The model under review builds one solid part; all positions refer to its coordinate system, in mm. Face numbers are marked on the shaded views. A direction names the side the tool comes from. Coordinates: 2 decimals unless noted, no trailing zeros. Order: outer loops, then holes, each group sorted by start corner. A loop starts at its lowest first (then second) coordinate and runs counter-clockwise, first axis right, second up. Notation, with made-up numbers: M 81,29.5 L 94,29.5 A15 cw 94,56.5 Z; hole C 85,69.25 d9. An arc over 180 degrees is marked long. Answer as CSV lines item,"result". Start each with the question number.
Q1. Wall thickness on L1, parallel to X at y = 0.8, z = 5; L2, parallel to X at y = 24.5, z = 3.75; L3, parallel to X at y = 26.6, z = 0: over which ranges is each line inside the solid? List them lowest first. Write a range as [from, to].
Q2. Consider section D-D on z = 0. Write out the cut boundary in (x, y).
Q3. Consider section C-C on y = 23. Write out the cut boundary in (x, z), and give its area (3 significant figures).
Q4. Consider section B-B on x = -24.3. Write out the cut boundary in (y, z), and give its area (3 significant figures).
Q5. Consider section A-A on x = 9.3. Write out the cut boundary in (y, z), and give its area (3 significant figures).
Q6. The part is to be moulded in two halves that separate along X. For the marked faces 1, 2, 3 and 4, say which applies: +X half, -X half, draft (parallel to the pull), parting line (faces both ways), or undercut.
Q7. Machinability: for the marked faces 5 and 6, which of the approach directions +Z, -Z, +X, -X, +Y, -Y give a long, thin tool a straight path to every point of the face, cutting with its end or side? Answer none if there is none.
Q8. For P1, Ø1.8, axis at x = -24.3, z = 5, coming from the -Y side; P2, Ø1.8, axis at x = -24.5, y = 3.5, coming from the -Z side; P3, Ø6.5, axis at x = 23, y = 5.5, coming from the +Z side, all flat-tipped, find the tip position at first contact; note any pin that passes through.
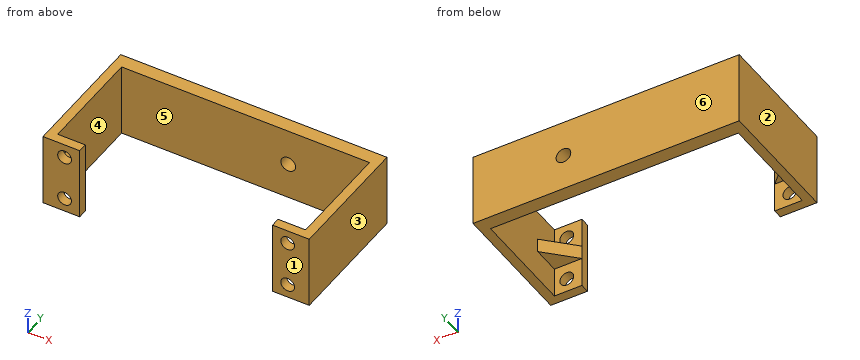
from build123d import *

# Parameters (mm, degrees)
RESSALTO_EXTRUS_O1_DEPTH = 8
ESBO_O2_R                = 1.5
CORTE_EXTRUS_O1_DEPTH    = 16
RESSALTO_EXTRUS_O3_DEPTH = 1.5
ESBO_O6_R                = 1.6
CORTE_EXTRUS_O2_DEPTH    = 3


with BuildPart() as part:
    # Esboço1 → Ressalto-extrusão1 (new, symmetric)
    with BuildSketch(Plane.XY):
        Polygon((-21, 0), (-29, 0), (-29, 28), (29, 28), (29, 0), (21, 0), (21, 2), (27, 2), (27, 25), (-27, 25), (-27, 2), (-21, 2), align=None)
    extrude(amount=RESSALTO_EXTRUS_O1_DEPTH, both=True)

    # Esboço2 → Corte-extrusão1 (cut)
    with BuildSketch(Plane.XZ):
        with Locations(Location((-24.3, -5, 0), (0, 0, 270))):
            Circle(ESBO_O2_R)
        with Locations(Location((-24.3, 5, 0), (0, 0, 270))):
            Circle(ESBO_O2_R)
        with Locations(Location((24.3, 5, 0), (0, 0, 270))):
            Circle(ESBO_O2_R)
        with Locations(Location((24.3, -5, 0), (0, 0, 270))):
            Circle(ESBO_O2_R)
    extrude(amount=-CORTE_EXTRUS_O1_DEPTH, mode=Mode.SUBTRACT)

    # Esboço4 → Ressalto-extrusão3 (add, symmetric)
    with BuildSketch(Plane.XY):
        Polygon((-21, 2), (-27, 8), (-27, 2), align=None)
        Polygon((21, 2), (27, 2), (27, 8), align=None)
    extrude(amount=RESSALTO_EXTRUS_O3_DEPTH, both=True)

    # Esboço6 → Corte-extrusão2 (cut)
    with BuildSketch(Plane(origin=(0, 28, 0), x_dir=(1, 0, 0), z_dir=(0, 1, 0))):
        with Locations(Location((9.3, 0, 0), (0, 0, 270))):
            Circle(ESBO_O6_R)
    extrude(amount=-CORTE_EXTRUS_O2_DEPTH, mode=Mode.SUBTRACT)


solid = part.part
Evaluation:
1,L1,"x = [-29, -25.8], [-22.8, -21], [21, 22.8], [25.8, 29]"
1,L2,"x = [-29, -27], [27, 29]"
1,L3,"x = [-29, 7.7], [10.9, 29]"
2,outline,"M -29,0 L -21,0 L -21,2 L -27,8 L -27,25 L 7.7,25 L 7.7,28 L -29,28 Z; M 10.9,25 L 27,25 L 27,8 L 21,2 L 21,0 L 29,0 L 29,28 L 10.9,28 Z"
3,outline,"M -29,-8 L -27,-8 L -27,8 L -29,8 Z; M 27,-8 L 29,-8 L 29,8 L 27,8 Z"
3,area,"64.0 mm²"
4,outline,"M 0,-8 L 2,-8 L 2,-6.5 L 0,-6.5 Z; M 0,-3.5 L 2,-3.5 L 2,-1.5 L 5.3,-1.5 L 5.3,1.5 L 2,1.5 L 2,3.5 L 0,3.5 Z; M 0,6.5 L 2,6.5 L 2,8 L 0,8 Z; M 25,-8 L 28,-8 L 28,8 L 25,8 Z"
4,area,"77.9 mm²"
5,outline,"M 25,-8 L 28,-8 L 28,-1.6 L 25,-1.6 Z; M 25,1.6 L 28,1.6 L 28,8 L 25,8 Z"
5,area,"38.4 mm²"
6,face 1,"draft"
6,face 2,"-X half"
6,face 3,"+X half"
6,face 4,"undercut"
7,face 5,"+Z, -Z"
7,face 6,"+Z, -Z, +X, -X, +Y"
8,P1,"stops at y = 25"
8,P2,"stops at z = -1.5"
8,P3,"stops at z = 1.5"
